Geometry: final body of the model. Coordinates: model frame, mm. Face numbers are marked on the shaded views. Give positions to 0.01 mm unless a question says otherwise; leave off trailing zeros. Write each loop counter-clockwise with the first axis right and the second up, starting at its lowest first coordinate (ties: lowest second). Pieces come first, ordered by that corner, then holes. Notation, with made-up numbers: (13.25, -37.75) -> (65.25, -37.75) arc R23 ccw to (65.25, -28.75) -> close; hole circle Ø4 at (-17, 11). An arc over 180 degrees is marked (long way). Answer in a Markdown table with one row per item. Add a question column.
Item 1: Draft query along Y for the marked faces 1, 2 and 3. Return one class per face: +Y half, -Y half, draft (parallel to the pull), parting line (faces both ways), or undercut.
Item 2: Section query C-C on z = 4.5. Output: boundary loops of the cut face in (x, y) (3 decimals), plus the area to 3 significant figures.
Item 3: Section query A-A on y = 0. Output: boundary loops of the cut face in (x, z) (3 decimals), plus the area to 3 significant figures.
Item 4: First-contact query: P1, Ø5, axis at x = 1, z = 1.5, coming from the +Y side; P2, Ø1, axis at x = -1.5, z = 10, coming from the +Y side; P3, Ø1, axis at x = -2.5, z = 2, coming from the -Y side; P4, Ø3, axis at y = 3.5, z = 10, coming from the -X side. Flat tips, straight axial feed; report the tip coordinate or a pass-through.
Item 5: Material intervals for probe 1 along Y at (x, z) = (0, 2.95) (3 decimals); probe 2 along Z at (x, y) = (0, 0); probe 3 along X at (y, z) = (1.5, 8.75), sorted ascending. Write a range as from..to.
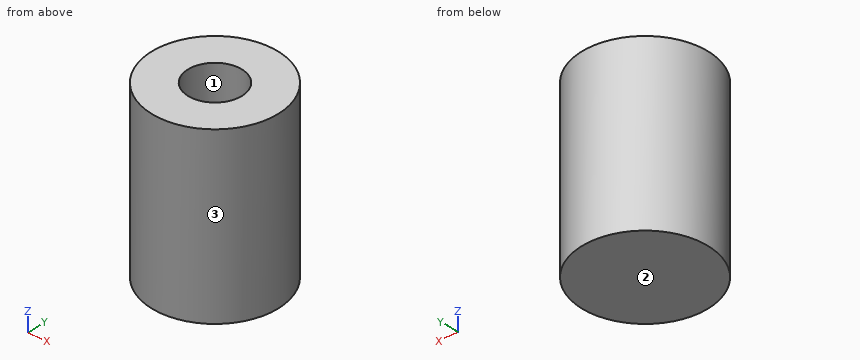
Autodesk Inventor part; units mm, degrees
ref_plane "YZ Plane" through (0, 0, 0) normal (1, 0, 0) x (0, 1, 0)
ref_plane "XZ Plane" through (0, 0, 0) normal (0, 1, 0) x (-1, 0, 0)
ref_plane "XY Plane" through (0, 0, 0) normal (0, 0, 1) x (1, 0, 0)
sketch "Boceto1" plane through (0, 0, 0) normal (0, 0, 1) x (1, 0, 0)
  circle A0 centre (0, 0) radius 4.75
  dimension "d0" = 9.5
extrude "Extrusión1" add sketch "Boceto1" along normal blind 13
sketch "Boceto2" plane through (0, 0, 13) normal (0, 0, 1) x (1, 0, 0)
  circle A0 centre (0, 0) radius 2.025
  dimension "d3" = 4.05
extrude "Extrusión2" cut sketch "Boceto2" against normal blind 11
sketch "Boceto3" plane through (0, 0, 0) normal (1, 0, 0) x (0, 1, 0)
  line L0 (2.025, 13) -> (2.025, 2)
  line L1 (2.025, 2) -> (2.025, 6)
  line L2 (1.25, 6) -> (-1.25, 6)
  line L3 (-2.025, 13) -> (-2.025, 2)
  line L4 (0, 6) -> (-1.25, 6)
  line L5 (0, 6) -> (1.25, 6)
  arc A0 (2.025, 6.775) -> (2.025, 5.225) centre (2.025, 6) ccw
  arc A1 (-2.025, 5.225) -> (-2.025, 6.775) centre (-2.025, 6) ccw
  line L6 (2.025, 6) -> (2.025, 10)
  line L7 (1.75, 10) -> (-1.75, 10)
  line L8 (0, 10) -> (-1.75, 10)
  line L9 (0, 10) -> (1.75, 10)
  arc A2 (2.025, 10.275) -> (2.025, 9.725) centre (2.025, 10) ccw
  arc A3 (-2.025, 9.725) -> (-2.025, 10.275) centre (-2.025, 10) ccw
  line L10 (-2.025, 2) -> (2.025, 2)
  line L11 (0, 2) -> (0, 13)
  line L12 (4.75, 13) -> (-4.75, 13)
  point P0 (0, 0)
  point P1 (2.025, 5.225)
  dimension "d7" = 4
  dimension "d8" = 1.25
  dimension "d9" = 1.25
  dimension "d10" = 4
  dimension "d11" = 1.75
  dimension "d12" = 1.75
revolve "Revolución1" add sketch "Boceto3" angle 360 about axis through (0, 0, 2) along (0, 0, 1) contours L0 A2 | A3 L3 | L0 A0 | A1 L3
properties part number "Cilindro_caucho" material "Caucho"
Findings below:
| question | item | result |
|---|---|---|
| 1 | face 1 | undercut |
| 1 | face 2 | draft |
| 1 | face 3 | parting line |
| 2 | outline | circle Ø9.5 at (0, 0); hole circle Ø4.05 at (0, 0) |
| 2 | area | 58.0 mm^2 |
| 3 | outline | (-4.75, 0) -> (4.75, 0) -> (4.75, 13) -> (2.025, 13) -> (2.025, 10.275) arc R0.275 ccw to (2.025, 9.725) -> (2.025, 6.775) arc R0.775 ccw to (2.025, 5.225) -> (2.025, 2) -> (-2.025, 2) -> (-2.025, 5.225) arc R0.775 ccw to (-2.025, 6.775) -> (-2.025, 9.725) arc R0.275 ccw to (-2.025, 10.275) -> (-2.025, 13) -> (-4.75, 13) -> close |
| 3 | area | 81.1 mm^2 |
| 4 | P1 | stops at y = 4.75 |
| 4 | P2 | stops at y = 4.64 |
| 4 | P3 | stops at y = -4.31 |
| 4 | P4 | stops at x = -4.31 |
| 5 | probe 1 | y = -4.75..-2.025, 2.025..4.75 |
| 5 | probe 2 | z = 0..2 |
| 5 | probe 3 | x = -4.51..-1.36, 1.36..4.51 |
